from build123d import *

# Parameters (mm, degrees)
SKETCH1_W            = 400
SKETCH1_H            = 150
BOSS_EXTRUDE1_DEPTH  = 6
SKETCH3_W            = 6
SKETCH3_H            = 25
CUT_EXTRUDE1_DEPTH   = 428.242320001
LPATTERN1_COUNT      = 2
LPATTERN1_PITCH      = 294
LPATTERN1_COUNT_DIR2 = 3
LPATTERN1_PITCH_DIR2 = 50
SKETCH4_W            = 6
SKETCH4_H            = 10
CUT_EXTRUDE2_DEPTH   = 428.242320001
LPATTERN2_COUNT      = 2
LPATTERN2_PITCH      = 258
LPATTERN2_COUNT_DIR2 = 2
LPATTERN2_PITCH_DIR2 = 140
SKETCH5_W            = 6
SKETCH5_H            = 10
CUT_EXTRUDE3_DEPTH   = 428.242320001
LPATTERN3_COUNT      = 2
LPATTERN3_PITCH      = 140
LPATTERN3_COUNT_DIR2 = 2
LPATTERN3_PITCH_DIR2 = 204


with BuildPart() as part:
    # Sketch1 → Boss-Extrude1 (new body)
    with BuildSketch(Plane(origin=(0, 0, 0), x_dir=(0, 0, -1), z_dir=(1, 0, 0))):
        with Locations((-200, 75)):
            Rectangle(SKETCH1_W, SKETCH1_H)
    extrude(amount=BOSS_EXTRUDE1_DEPTH)

    # Sketch3 → Cut-Extrude1 (cut, through all)
    with BuildSketch(Plane(origin=(6, 0, 0), x_dir=(0, 0, -1), z_dir=(1, 0, 0))):
        with Locations((-347, 137.5)):
            Rectangle(SKETCH3_W, SKETCH3_H)
    cut_extrude1 = extrude(amount=-CUT_EXTRUDE1_DEPTH, mode=Mode.SUBTRACT)

    # LPattern1: Cut-Extrude1 2 × 3
    with Locations(*[(0, -j * LPATTERN1_PITCH_DIR2, -i * LPATTERN1_PITCH) for i in range(LPATTERN1_COUNT) for j in range(LPATTERN1_COUNT_DIR2) if (i, j) != (0, 0)]):
        add(cut_extrude1, mode=Mode.SUBTRACT)

    # Sketch4 → Cut-Extrude2 (cut, through all)
    with BuildSketch(Plane(origin=(6, 0, 0), x_dir=(0, 0, -1), z_dir=(1, 0, 0))):
        with Locations((-329, 145)):
            Rectangle(SKETCH4_W, SKETCH4_H)
    cut_extrude2 = extrude(amount=-CUT_EXTRUDE2_DEPTH, mode=Mode.SUBTRACT)

    # LPattern2: Cut-Extrude2 2 × 2
    with Locations(*[(0, -j * LPATTERN2_PITCH_DIR2, -i * LPATTERN2_PITCH) for i in range(LPATTERN2_COUNT) for j in range(LPATTERN2_COUNT_DIR2) if (i, j) != (0, 0)]):
        add(cut_extrude2, mode=Mode.SUBTRACT)

    # Sketch5 → Cut-Extrude3 (cut, through all)
    with BuildSketch(Plane(origin=(6, 0, 0), x_dir=(0, 0, -1), z_dir=(1, 0, 0))):
        with Locations((-299, 145)):
            Rectangle(SKETCH5_W, SKETCH5_H)
    cut_extrude3 = extrude(amount=-CUT_EXTRUDE3_DEPTH, mode=Mode.SUBTRACT)

    # LPattern3: Cut-Extrude3 2 × 2
    with Locations(*[(0, -i * LPATTERN3_PITCH, -j * LPATTERN3_PITCH_DIR2) for i in range(LPATTERN3_COUNT) for j in range(LPATTERN3_COUNT_DIR2) if (i, j) != (0, 0)]):
        add(cut_extrude3, mode=Mode.SUBTRACT)


solid = part.part
Could you check a few things on this model? Use its own coordinates, in mm. Give positions to 0.01 mm unless a question says otherwise; leave off trailing zeros. Write each loop counter-clockwise with the first axis right and the second up, starting at its lowest first coordinate (ties: lowest second). Pieces come first, ordered by that corner, then holes. Notation, with made-up numbers: (-31.75, -11) -> (-2.75, -11) arc R18 ccw to (-2.75, 21) -> close; hole circle Ø1 at (67, 21.5). An arc over 180 degrees is marked (long way). Answer as CSV lines item,"result". Start each with the question number.
(1) If we section it at A-A, the plane y = 82.5: Write out the boundary of the cut face in (x, z), and give its area (3 significant figures).
(2) Please list where these lines run through material, in increasing order: line 1 (Z direction, x = 3.3, y = 26); line 2 (Y direction, x = 5.4, z = 346).
(3) If we section it at B-B, the plane x = 5.05: Give the number of separate pieces and of enclosed holes in the cut face, and give its area (3 significant figures).
(4) I'm going to push flat-ended pins straight in: pin 1 Ø3 at (x, y) = (3.5, 146) entering from -Z; pin 2 Ø3 at (x, z) = (2, 348) entering from +Y; pin 3 Ø3 at (x, z) = (4.5, 300) entering from -Y; pin 4 Ø1.8 at (x, z) = (2, 72) entering from +Y. Where does each tip first touch, or does it pass through?
Answer list:
1,outline,"(0, 0) -> (6, 0) -> (6, 50) -> (0, 50) -> close; (0, 56) -> (6, 56) -> (6, 344) -> (0, 344) -> close; (0, 350) -> (6, 350) -> (6, 400) -> (0, 400) -> close"
1,area,"2,330 mm^2"
2,line 1,"0 to 50, 56 to 344, 350 to 400"
2,line 2,"0 to 25, 50 to 75, 100 to 125"
3,separate pieces,"1"
3,enclosed holes,"4"
3,area,"58,600 mm^2"
4,pin 1,"z = 0"
4,pin 2,"y = 125"
4,pin 3,"y = 10"
4,pin 4,"y = 140"
